Autodesk Inventor part; units mm, degrees
ref_plane "YZ Plane" through (0, 0, 0) normal (1, 0, 0) x (0, 1, 0)
ref_plane "XZ Plane" through (0, 0, 0) normal (0, 1, 0) x (-1, 0, 0)
ref_plane "XY Plane" through (0, 0, 0) normal (0, 0, 1) x (1, 0, 0)
sketch "Sketch1" plane through (0, 0, 0) normal (0, 1, 0) x (-1, 0, 0)
  line L0 (6, 11.5) -> (-6, 11.5)
  line L1 (-6, 11.5) -> (-6, -11.5)
  line L2 (-6, -11.5) -> (6, -11.5)
  line L3 (6, -11.5) -> (6, 11.5)
  line L4 (6, 11.5) -> (-6, -11.5) construction
  line L5 (-6, 11.5) -> (6, -11.5) construction
  point P0 (0, 0)
  dimension "d0" = 12
  dimension "d1" = 23
extrude "Extrusion1" add sketch "Sketch1" along normal mid plane 22.5
sketch "Sketch2" plane through (-6, 11.25, 11.5) normal (0, 0, 1) x (1, 0, 0)
  line L0 (12, -22.5) -> (0, -22.5)
  line L1 (0, -22.5) -> (0, 0)
  line L2 (0, -6.5) -> (12, -6.5)
  line L3 (12, -22.5) -> (12, 0)
  line L4 (0, -4.2) -> (12, -4.2)
  line L5 (0, -4.2) -> (0, -6.5)
  line L6 (12, -4.2) -> (12, -6.5)
  point P0 (6, -11.25)
  dimension "d4" = 16
  dimension "d5" = 2.3
extrude "Extrusion2" add sketch "Sketch2" along normal blind 4.5 contours L2 L1 L4 L3
mirror "Mirror1" about plane through (0, 0, 0) normal (0, 0, 1) of "Extrusion2"
sketch "Sketch3" plane through (-6, 7.05, 11.5) normal (0, 1, 0) x (1, 0, 0)
  arc A0 (6.5, -3.804) -> (5.5, -3.804) centre (6, -2.55) ccw
  line L0 (0, 0) -> (0, -4.5)
  line L1 (12, -4.5) -> (0, -4.5) construction
  line L2 (6, -2.55) -> (6, -4.5) construction
  line L3 (0, -4.5) -> (12, -4.5) construction
  line L4 (6, -2.55) -> (6, -1.2) construction
  line L5 (5.5, -4.5) -> (5.5, -3.804)
  line L6 (6.5, -4.5) -> (6.5, -3.804)
  line L7 (6.5, -4.5) -> (5.5, -4.5)
  point P0 (6, 11.5)
  point P1 (5.5, -2.8875)
  point P2 (6.5, -2.8875)
  dimension "d8" = 2.7
  dimension "d9" = 6
  dimension "d11" = 0.5
  dimension "d14" = 1.95
extrude "Extrusion3" cut sketch "Sketch3" against normal blind 4.5
mirror "Mirror2" about plane through (0, 0, 0) normal (0, 0, 1) of "Extrusion3"
sketch "Sketch4" plane through (0, 11.25, 0) normal (0, 1, 0) x (1, 0, 0)
  circle A0 centre (0, -5.5) radius 6
  line L0 (-6, 11.5) -> (-6, -11.5)
  line L1 (-6, -11.5) -> (6, -11.5)
  circle A1 centre (0, -5.5) radius 2.5
  point P0 (0, 0)
  dimension "d17" = 5
extrude "Extrusion4" add sketch "Sketch4" along normal blind 4 contours A0
sketch "Sketch5" plane through (0, 11.25, 0) normal (0, 1, 0) x (1, 0, 0)
  circle A0 centre (0, 0.75) radius 2.5
  circle A1 centre (0, -5.5) radius 2.5
  point P0 (0, 0)
  dimension "d20" = 5
  dimension "d21" = 6.25
extrude "Extrusion5" add sketch "Sketch5" along normal blind 4 contours A0
sketch "Sketch6" plane through (0, 11.25, 5.5) normal (0, 1, 0) x (1, 0, 0)
  circle A0 centre (0, 0) radius 2.5
  point P0 (0, 5.5)
extrude "Extrusion6" cut sketch "Sketch6" against normal blind 10
properties part number "Servo body"
Geometry check sheet. Reference: the model listing, model coordinates, mm. A direction names the side the tool comes from. Coordinates: 2 decimals unless noted, no trailing zeros. Order: outer loops, then holes, each group sorted by start corner. A loop starts at its lowest first (then second) coordinate and runs counter-clockwise, first axis right, second up. Notation, with made-up numbers: (39, -11.5) - (84, -11.5) arc R10 ccw to (84, 6.5) - close; hole circle Ø10 at (-30, 62). An arc over 180 degrees is marked (long way). One line per item, written item: value.
(1) Access from +Z, -Z, +X, -X, +Y, -Y to the whole of each face (thin tool, end or side, straight path). Record for faces 4 (the face through (1.4, 7.05, -13.2)), 5 (the face through (0, -3, -11.5)), 6 (the face through (0, 1.25, 5)), 7 (the face through (0, 11.25, -5)), 8 (the face through (0, 9, 11.5)).
Data:
face 4: -Z, +X, -X, +Y
face 5: -Z, +X, -X, -Y
face 6: +Y
face 7: -Z, +Y
face 8: +Z, +X, -X, +Y
(2) Sectioned sample at B-B (z = 14.05). Enter the section's corners in (x, y).
Data:
outline: (-6, 4.75) - (-1.35, 4.75) - (-1.35, 7.05) - (-6, 7.05) - close; (1.35, 4.75) - (6, 4.75) - (6, 7.05) - (1.35, 7.05) - close
(3) Sectioned sample at A-A (y = 6). Enter the section's corners in (x, z), and give its area (3 significant figures).
Data:
outline: (-6, -16) - (-0.5, -16) - (-0.5, -15.3) arc R1.35 cw (long way) to (0.5, -15.3) - (0.5, -16) - (6, -16) - (6, 16) - (0.5, 16) - (0.5, 15.3) arc R1.35 cw (long way) to (-0.5, 15.3) - (-0.5, 16) - (-6, 16) - close; hole circle Ø5 at (0, 5.5)
area: 352 mm^2
(4) Release check for a two-part mould opening along Z. For faces 1 (the face through (3, 6, -16)), 2 (the face through (5, 11.25, 10)), 3 (the face through (-0.07, 13.22, -3.25)) record: +Z half, -Z half, draft (parallel to the pull), parting line (faces both ways), or undercut.
Data:
face 1: -Z half
face 2: draft
face 3: undercut
(5) Sectioned sample at D-D (y = -0.5). Enter the section's corners in (x, z).
Data:
outline: (-6, -11.5) - (6, -11.5) - (6, 11.5) - (-6, 11.5) - close
(6) Sectioned sample at C-C (z = -0.75). Enter the section's corners in (x, y).
Data:
outline: (-6, -11.25) - (6, -11.25) - (6, 11.25) - (2.5, 11.25) - (2.5, 15.25) - (-2.5, 15.25) - (-2.5, 11.25) - (-6, 11.25) - close
(7) Depth check by flat-ended pin: pin 1 Ø1.3 at (x, z) = (2.5, -14) entering from +Y; pin 2 Ø5 at (x, z) = (2.5, 14.5) entering from -Y; pin 3 Ø1.3 at (x, y) = (-2.5, 9) entering from -Z. Enter the tip coordinate at first touch or a pass-through.
Data:
pin 1: stops at y = 7.05
pin 2: stops at y = 4.75
pin 3: stops at z = -11.5
(8) Thickness scan on probe 1 along X at (y, z) = (12, 5.5); probe 2 along Z at (x, y) = (0, 6.5); probe 3 along X at (y, z) = (5.65, -14.05). Record the ranges inside material, lowest first. Write a range as from..to.
Data:
probe 1: x = -6..-2.5, 2.5..6
probe 2: z = -12.7..3, 8..12.7
probe 3: x = -6..-1.35, 1.35..6
